from build123d import *

# Parameters (mm, degrees)
SKETCH1_R                      = 41.275
BOSS_EXTRUDE1_DEPTH            = 59.436
CUT_EXTRUDE5_START             = -54.356
SKETCH7_R                      = 41.275
SKETCH7_R_2                    = 34.925
CUT_EXTRUDE5_DEPTH             = 54.356
TOP_INTERCONNECTION_HOLE_REACH = 85.306
SKETCH8_R                      = 2.413
CIRPATTERN1_COUNT              = 6
SKETCH9_R                      = 32.385
CUT_EXTRUDE8_DEPTH             = 10.16


with BuildPart() as part:
    # Sketch1 → Boss-Extrude1 (new body)
    with BuildSketch(Plane(origin=(0, 0, 0), x_dir=(1, 0, 0), z_dir=(0, 1, 0))):
        with Locations(Location((0, 0, 0), (0, 0, 270))):
            Circle(SKETCH1_R)
    extrude(amount=-BOSS_EXTRUDE1_DEPTH)

    # Sketch7 → Cut-Extrude5 (cut)
    with BuildSketch(Plane.XZ.offset(59.436).offset(CUT_EXTRUDE5_START)):
        with Locations(Location((0, 0, 0), (0, 0, 90))):
            Circle(SKETCH7_R)
        with Locations(Location((0, 0, 0), (0, 0, 270))):
            Circle(SKETCH7_R_2, mode=Mode.SUBTRACT)
    extrude(amount=CUT_EXTRUDE5_DEPTH, mode=Mode.SUBTRACT)

    # Sketch8 → Top Interconnection Hole (cut, up to next)
    with BuildSketch(Plane(origin=(0, 0, 0), x_dir=(1, 0, 0), z_dir=(0, 1, 0)), mode=Mode.PRIVATE) as top_interconnection_hole_sk1:
        with Locations(Location((-36.83, 0, 0), (0, 0, 270))):
            Circle(SKETCH8_R)
    top_interconnection_hole_tool1 = extrude(top_interconnection_hole_sk1.sketch, amount=-TOP_INTERCONNECTION_HOLE_REACH, mode=Mode.PRIVATE) & part.part
    top_interconnection_hole = top_interconnection_hole_tool1.solids().sort_by_distance((-36.83, 0, 0))[0]
    add(top_interconnection_hole, mode=Mode.SUBTRACT)

    # CirPattern1: Top Interconnection Hole ×6 about axis
    cirpattern1_axis = Axis((0, 0, 0), (0, 1, 0))
    for i in range(1, CIRPATTERN1_COUNT):
        add(top_interconnection_hole.rotate(cirpattern1_axis, i * 360 / CIRPATTERN1_COUNT), mode=Mode.SUBTRACT)

    # Sketch9 → Cut-Extrude8 (cut)
    with BuildSketch(Plane(origin=(0, 0, 0), x_dir=(1, 0, 0), z_dir=(0, 1, 0))):
        with Locations(Location((0, 0, 0), (0, 0, 270))):
            Circle(SKETCH9_R)
    extrude(amount=-CUT_EXTRUDE8_DEPTH, mode=Mode.SUBTRACT)


solid = part.part
Input: part model. Units: mm. Frame: model coordinates. A direction names the side the tool comes from. Give positions to 0.01 mm unless a question says otherwise; leave off trailing zeros. Order: outer loops, then holes, each group sorted by start corner. A loop starts at its lowest first (then second) coordinate and runs counter-clockwise, first axis right, second up.
Q1. Contact query for flat-ended pins moving along their axis: pin 1 Ø1 at (x, z) = (-18.5, 19.5) entering from +Y; pin 2 Ø1.5 at (x, y) = (6.5, -35) entering from -Z; pin 3 Ø6.5 at (x, z) = (-18.42, 31.9) entering from +Y; pin 4 Ø2 at (y, z) = (-29.5, -1.5) entering from +X. Output: stop coordinate, or through.
Checked values:
pin 1: stops at y = -10.16
pin 2: stops at z = -34.45
pin 3: stops at y = 0
pin 4: stops at x = 34.9
Q2. Section C-C on y = -40. Output: boundary loops of the cut face in (x, z) (3 decimals), and give its area (3 significant figures).
Checked values:
outline: (-34.895, -1.442) arc R34.925 ccw to (-18.696, -29.499) arc R2.413 cw to (-16.199, -30.941) arc R34.925 ccw to (16.199, -30.941) arc R2.413 cw to (18.696, -29.499) arc R34.925 ccw to (34.895, -1.442) arc R2.413 cw to (34.895, 1.442) arc R34.925 ccw to (18.696, 29.499) arc R2.413 cw to (16.199, 30.941) arc R34.925 ccw to (-16.199, 30.941) arc R2.413 cw to (-18.696, 29.499) arc R34.925 ccw to (-34.895, 1.442) arc R2.413 cw to start
area: 3,830 mm2
Q3. Ray query, probe 1 along Y at (x, z) = (10.5, -28); probe 2 along X at (y, z) = (-12.5, -13); probe 3 along Y at (x, z) = (16, -35). Return the intervals inside material, ascending.
Checked values:
probe 1: y = -59.44 to -10.16
probe 2: x = -32.42 to 32.42
probe 3: y = -5.08 to 0
Q4. Draft query along X for faces 1 (the cylindrical face through (-0.236, -31.878, -34.924)), 2 (the cylindrical face through (34.6, -22.98, 0.92)), 3 (the flat face through (-34, -5.08, -9)), 4 (the cylindrical face through (30.127, -31.878, -17.666)). Return one class per face: +X half, -X half, draft (parallel to the pull), parting line (faces both ways), or undercut.
Checked values:
face 1: parting line
face 2: undercut
face 3: draft
face 4: +X half
Q5. Set-up query: faces 5 (the flat face through (0, -10.16, 0)), 6 (the cylindrical face through (30.36, -31.88, 17.26)), 7 (the cylindrical face through (-30.36, -31.88, -17.26)), 8 (the cylindrical face through (0.236, -31.878, 34.924)), 9 (the cylindrical face through (-30.127, -31.878, 17.666)). Return all of +Z, -Z, +X, -X, +Y, -Y with unobstructed straight access to the full face (end or side cutting, diameter ignored); none if empty.
Checked values:
face 5: +Y
face 6: +Z, +X, -Y
face 7: -Z, -X, -Y
face 8: +Z, -Y
face 9: +Z, -X, -Y
Q6. Section D-D on x = -36.83. Output: boundary loops of the cut face in (y, z).
Checked values:
outline: (-5.08, -18.63) - (0, -18.63) - (0, -2.41) - (-5.08, -2.41) - close; (-5.08, 2.41) - (0, 2.41) - (0, 18.63) - (-5.08, 18.63) - close
Q7. Section A-A on z = 0. Output: boundary loops of the cut face in (x, y) (3 decimals), and give its area (3 significant figures).
Checked values:
outline: (-41.275, -5.08) - (-39.243, -5.08) - (-39.243, 0) - (-41.275, 0) - close; (-34.417, -59.436) - (34.417, -59.436) - (34.417, 0) - (32.385, 0) - (32.385, -10.16) - (-32.385, -10.16) - (-32.385, 0) - (-34.417, 0) - close; (39.243, -5.08) - (41.275, -5.08) - (41.275, 0) - (39.243, 0) - close
area: 3,450 mm2
Q8. Section B-B on x = 0. Output: boundary loops of the cut face in (y, z) (3 decimals).
Checked values:
outline: (-59.436, -34.925) - (-5.08, -34.925) - (-5.08, -41.275) - (0, -41.275) - (0, -32.385) - (-10.16, -32.385) - (-10.16, 32.385) - (0, 32.385) - (0, 41.275) - (-5.08, 41.275) - (-5.08, 34.925) - (-59.436, 34.925) - close
